Geometry check sheet. Reference: drawing and pictorial views, mm from the part's lowest x, y, z. Round coordinates to 2 decimals unless told otherwise and drop trailing zeros. Loops run counter-clockwise (first coordinate to the right, second up) from the corner with the lowest first, then second, coordinate; pieces in that order, holes last. Notation, with made-up numbers: (63.25, 13) - (69.25, 13) arc R10 ccw to (69.25, 23) - close; hole circle Ø2 at (41, 40). An arc over 180 degrees is marked (long way). Put each result on its own line as item: value. Start each with the question number.
Item 1: Gauge pin test, flat end, axial feed: pin 1 Ø1 at (x, z) = (262, 317) entering from -Y. Record the tip position at first contact, or that the pin passes through.
Item 2: Section check B-B, the plane z = 178.5. Record the cut outline in (x, y).
Item 3: Section check C-C, the plane x = 59. Record the cut outline in (y, z).
Item 4: Section check A-A, the plane y = 25.5. Record the cut outline in (x, z), and give its area (3 significant figures).
Item 5: Draft check along X on the marked faces 1, 2, 3 and 4. Enter one of: pulls with the +X half, pulls with the -X half, needs draft (parallel to the pull), parting line crosses it, or undercut.
Item 6: Material ranges on line 1 along X through (y, z) = (138.5, 144.5); line 2 along Y through (x, z) = (94, 336), recorded low to high.
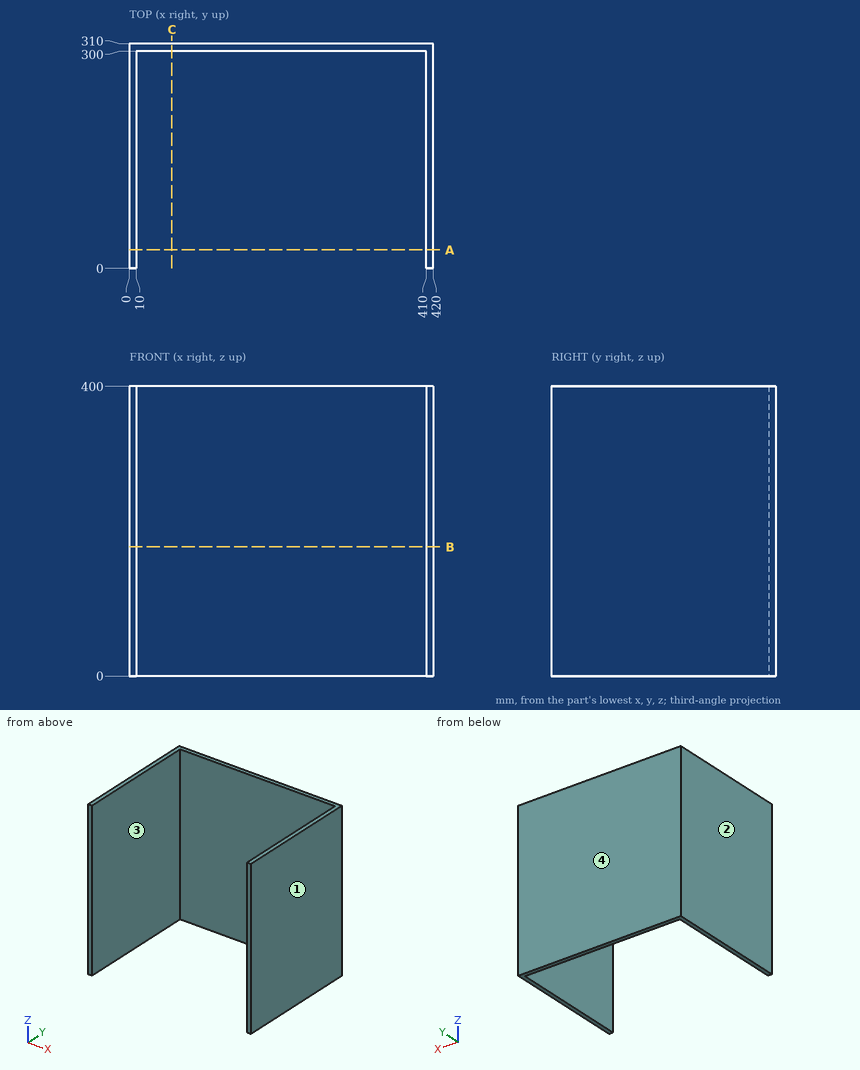
Check result:
1. pin 1: y = 300
2. outline: (0, 0) - (10, 0) - (10, 300) - (410, 300) - (410, 0) - (420, 0) - (420, 310) - (0, 310) - close
3. outline: (300, 0) - (310, 0) - (310, 400) - (300, 400) - close
4. outline: (0, 0) - (10, 0) - (10, 400) - (0, 400) - close; (410, 0) - (420, 0) - (420, 400) - (410, 400) - close
4. area: 8,000 mm²
5. face 1: pulls with the +X half
5. face 2: pulls with the -X half
5. face 3: undercut
5. face 4: needs draft
6. line 1: 0 to 10, 410 to 420
6. line 2: 300 to 310
